Geometry check sheet. Reference: the model listing, model coordinates, mm. Face numbers are marked on the shaded views. A direction names the side the tool comes from. Round coordinates to 2 decimals unless told otherwise and drop trailing zeros. Write each loop counter-clockwise with the first axis right and the second up, starting at its lowest first coordinate (ties: lowest second). Pieces come first, ordered by that corner, then holes.
Item 1: Cross-section at B-B (x = -39.5). Enter the section's corners in (y, z), then the cut area to 3 significant figures.
Item 2: Cross-section at A-A (z = 15). Enter the section's corners in (x, y).
Item 3: Scan lines: probe 1 along Y at (x, z) = (-33, 10); probe 2 along X at (y, z) = (29.5, 14.5); probe 3 along Y at (x, z) = (-22, 24). Record each from-to range of solid material in increasing order.
Item 4: Draft check along X on the marked faces 3, 4 and 5. Enter one of: pulls with the +X half, pulls with the -X half, needs draft (parallel to the pull), parting line crosses it, or undercut.
Item 5: Cross-section at C-C (y = 37). Enter the section's corners in (x, z).
Item 6: Depth check by flat-ended pin: P1, Ø10, axis at y = 30.5, z = 44.5, coming from the +X side; P2, Ø11.5, axis at x = -27.5, z = 18.5, coming from the +Y side; P3, Ø1, axis at x = -37, z = 31.5, coming from the +Y side; P4, Ø4, axis at x = -25, z = 23.5, coming from the -Y side. Enter the tip coordinate at first touch or a pass-through.
Item 7: Cross-section at D-D (x = -7.5). Enter the section's corners in (y, z).
Item 8: Access from +Z, -Z, +X, -X, +Y, -Y to the whole of each face (thin tool, end or side, straight path). Record for the marked faces 1 and 2.
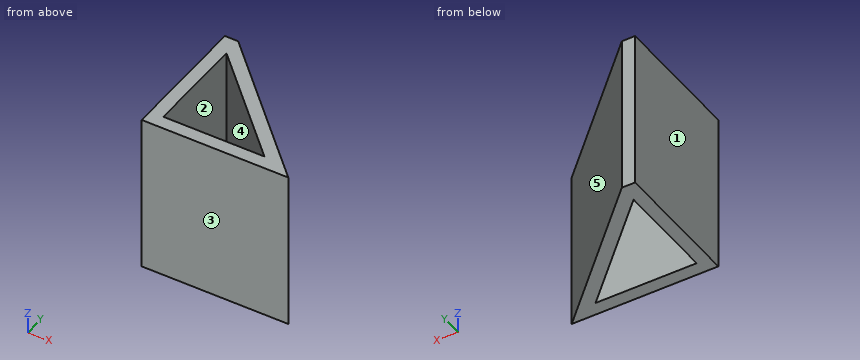
from build123d import *

# Parameters (mm, degrees)
F1_DEPTH = 60


with BuildPart() as f1:
    # F0 (on Top) → F1 (new body)
    with BuildSketch(Plane.XY):
        Polygon((-55, 0), (0, 0), (-50, 50), (-55, 50), align=None)
        Polygon((-50, 5), (-50, 42.928932), (-12.071068, 5), align=None, mode=Mode.SUBTRACT)
    extrude(amount=F1_DEPTH)


solid = f1.part
Resolved:
1. outline: (0, 0) - (5, 0) - (5, 60) - (0, 60) - close; (32.43, 0) - (39.5, 0) - (39.5, 60) - (32.43, 60) - close
1. area: 724 mm2
2. outline: (-55, 0) - (0, 0) - (-50, 50) - (-55, 50) - close; hole (-50, 5) - (-12.07, 5) - (-50, 42.93) - close
3. probe 1: y = 0 to 5, 25.93 to 33
3. probe 2: x = -55 to -50, -36.57 to -29.5
3. probe 3: y = 0 to 5, 14.93 to 22
4. face 3: needs draft
4. face 4: undercut
4. face 5: pulls with the +X half
5. outline: (-55, 0) - (-50, 0) - (-50, 60) - (-55, 60) - close; (-44.07, 0) - (-37, 0) - (-37, 60) - (-44.07, 60) - close
6. P1: stops at x = -25.5
6. P2: stops at y = 33.25
6. P3: stops at y = 37.5
6. P4: stops at y = 0
7. outline: (0, 0) - (7.5, 0) - (7.5, 60) - (0, 60) - close
8. face 1: +Z, -Z, -X, +Y, -Y
8. face 2: +Z, -Z
